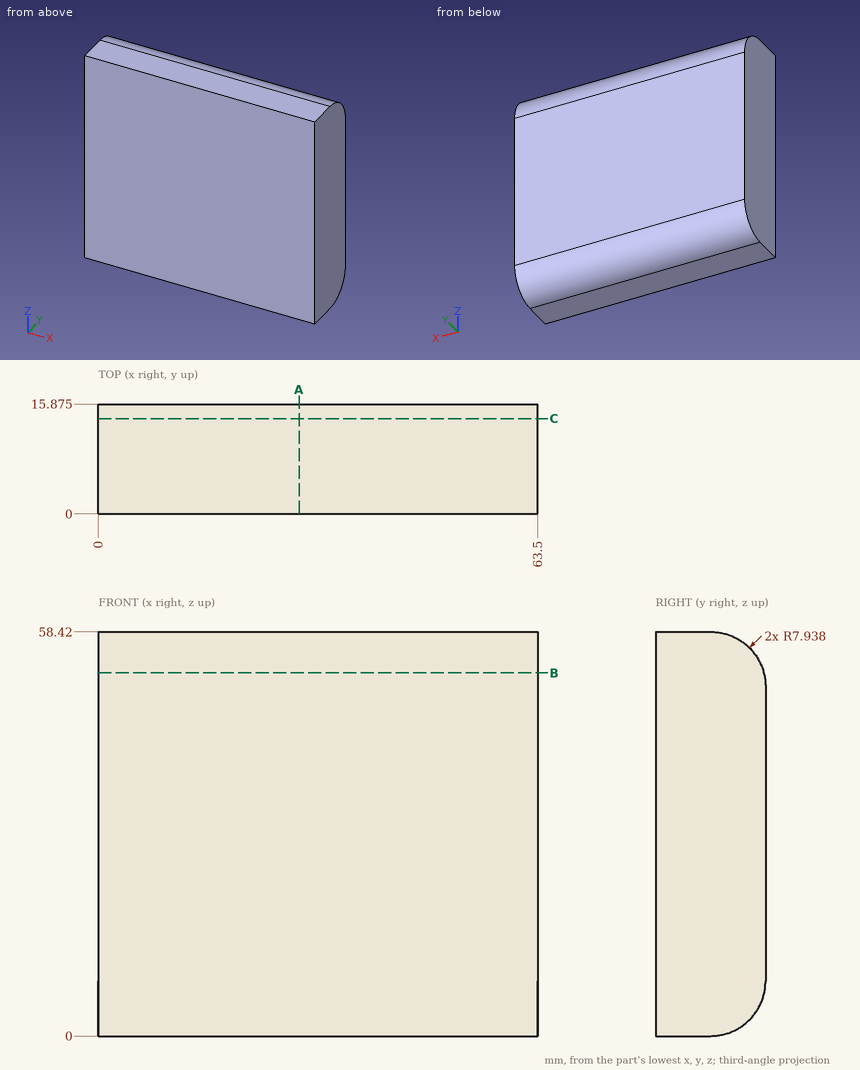
Study the drawing (mm; zero at the part's minimum x, y, z) and answer. Give positions to 0.01 mm unless a question says otherwise; leave off trailing zeros. Write each loop counter-clockwise with the first axis right and the second up, starting at its lowest first coordinate (ties: lowest second). Pieces come first, ordered by that corner, then holes.
Item 1: Find the intervals of material crossed by line 1 along Y through (x, z) = (24.5, 55.5); line 2 along Y through (x, z) = (57.5, 4.5); line 3 along Z through (x, y) = (7, 9.5) (1 decimal), in increasing order.
Item 2: Section A-A, the plane x = 29 is taken. Write down the section's boundary in (y, z) (1 decimal).
Item 3: A flat-ended cylindrical pin translates along its axis: P1, Ø6, axis at x = 49, y = 12, coming from the +Z side. Find the tip coordinate at first contact, or state that the pin passes through.
Item 4: Section C-C, the plane y = 13.75 is taken. Write down the section's boundary in (x, z).
Item 5: Section B-B, the plane z = 52.5 is taken. Write down the section's boundary in (x, y) (1 decimal).
Completed:
1. line 1: y = 0 to 14.09
1. line 2: y = 0 to 15.09
1. line 3: z = 0.2 to 58.3
2. outline: (0, 0) - (7.9, 0) arc R7.9 ccw to (15.9, 7.9) - (15.9, 50.5) arc R7.9 ccw to (7.9, 58.4) - (0, 58.4) - close
3. P1: stops at z = 58.35
4. outline: (0, 2.53) - (63.5, 2.53) - (63.5, 55.89) - (0, 55.89) - close
5. outline: (0, 0) - (63.5, 0) - (63.5, 15.6) - (0, 15.6) - close
